Geometry check sheet. Reference: the model listing, model coordinates, mm. A direction names the side the tool comes from. Give positions to 0.01 mm unless a question says otherwise; leave off trailing zeros. Order: outer loops, then holes, each group sorted by start corner. A loop starts at its lowest first (then second) coordinate and runs counter-clockwise, first axis right, second up. Notation, with made-up numbers: M 54.25,-21 L 64.25,-21 A6 cw 64.25,-15 Z; hole C 60.25,27 d11. An arc over 180 degrees is marked long. Put each result on its own line as item: value. Start each with the question number.
Q1. Access from +Z, -Z, +X, -X, +Y, -Y to the whole of each face (thin tool, end or side, straight path). Record for faces 1 (the flat face through (-40, 0, 13)), 2 (the flat face through (-41, 25, 19.05)), 3 (the cylindrical face through (-39.92, 1.91, 23.59)), 4 (the cylindrical face through (-40.49, 48.89, -23.59)).
Q2. Go/stop test with flat-tipped pins: pin 1 (11.5 mm diameter, centred on x = -40.5, y = 18.5, fed in from -Z); pin 2 (3 mm diameter, centred on x = -23, y = 39, fed in from +Z); pin 3 (23 mm diameter, centred on x = 26.67, z = -0.23, fed in from -Y); pin 4 (6.5 mm diameter, centred on y = 27.5, z = 31.5, fed in from -X). Record where each tip stops, or that it passes through.
Q3. Material ranges on L1, parallel to Y at x = 38, z = -29; L2, parallel to Z at x = -50.5, y = 12, recorded low to high.
Q4. Section check B-B on x = 26.67. Record the cut outline in (y, z), then the cut area to 3 significant figures.
Q5. Section check D-D on x = -21.5. Record the cut outline in (y, z), then the cut area to 3 significant figures.
Q6. Mould release check, pull along Z, two halves, no side actions. Record for faces 5 (the flat face through (-40, 50.8, -13)), 6 (the flat face through (-0.4, 26.8, 38.1)), 7 (the cylindrical face through (13.982, 56.471, 0.333)): +Z half, -Z half, draft (parallel to the pull), parting line (faces both ways), or undercut.
Q7. Section check A-A on y = 14. Record the cut outline in (x, z).
Q8. Section check C-C on z = 31. Record the cut outline in (x, y), then the cut area to 3 significant figures.
```python
from build123d import *

# Parameters (mm, degrees)
F1_DEPTH      = 38.1
F2_R          = 12.7
F3_DEPTH      = 59.6909986267
F3_DEPTH_BACK = 25.4
F4_W          = 38.0999967456
F4_H          = 38.0999967456
F5_DEPTH      = 76.2
F6_R          = 12.7
F7_DEPTH      = 59.6909987267


with BuildPart() as f1:
    # F0 (on Top) → F1 (new body, symmetric)
    with BuildSketch(Plane.XY):
        with BuildLine():
            Line((46.99, 59.6899986267), (6.35, 59.6899986267))
            ThreePointArc((6.35, 59.6899986267), (-2.63025515, 55.97025515), (-6.3499986267, 46.99))
            Line((-6.3499986267, 46.99), (-6.3499986267, 6.35))
            ThreePointArc((-6.3499986267, 6.35), (-2.63025515, -2.63025515), (6.35, -6.3499986267))
            Line((6.35, -6.3499986267), (46.99, -6.3499986267))
            ThreePointArc((46.99, -6.3499986267), (55.97025515, -2.63025515), (59.6899986267, 6.35))
            Line((59.6899986267, 6.35), (59.6899986267, 46.99))
            ThreePointArc((59.6899986267, 46.99), (55.97025515, 55.97025515), (46.99, 59.6899986267))
        make_face()
        with BuildLine():
            Line((46.99, 0), (6.35, 0))
            ThreePointArc((6.35, 0), (1.8598719395, 1.8598719395), (0, 6.35))
            Line((0, 6.35), (0, 46.99))
            ThreePointArc((0, 46.99), (1.8598719395, 51.4801280605), (6.35, 53.34))
            Line((6.35, 53.34), (46.99, 53.34))
            ThreePointArc((46.99, 53.34), (51.4801280605, 51.4801280605), (53.34, 46.99))
            Line((53.34, 46.99), (53.34, 6.35))
            ThreePointArc((53.34, 6.35), (51.4801280605, 1.8598719395), (46.99, 0))
        make_face(mode=Mode.SUBTRACT)
    extrude(amount=F1_DEPTH, both=True)

    # F2 (on Front) → F3 (cut, two sides)
    with BuildSketch(Plane.XZ) as f3_sk:
        with Locations((26.67, -0.2257099867)):
            Circle(F2_R)
    extrude(amount=-F3_DEPTH, mode=Mode.SUBTRACT)
    extrude(f3_sk.sketch, amount=F3_DEPTH_BACK, mode=Mode.SUBTRACT)

    # F4 (on Right) → F5 (join)
    with BuildSketch(Plane.YZ):
        with BuildLine():
            ThreePointArc((50.8, 19.05), (48.9401280605, 23.5401280605), (44.45, 25.4))
            Line((44.45, 25.4), (6.35, 25.4))
            ThreePointArc((6.35, 25.4), (1.8598719395, 23.5401280605), (0, 19.05))
            Line((0, 19.05), (0, -19.05))
            ThreePointArc((0, -19.05), (1.8598719395, -23.5401280605), (6.35, -25.4))
            Line((6.35, -25.4), (44.45, -25.4))
            ThreePointArc((44.45, -25.4), (48.9401280605, -23.5401280605), (50.8, -19.05))
            Line((50.8, -19.05), (50.8, 19.05))
        make_face()
        with Locations((25.4, 0)):
            Rectangle(F4_W, F4_H, mode=Mode.SUBTRACT)
    extrude(amount=-F5_DEPTH)

    # F6 (on Front) → F7 (cut, through all)
    with BuildSketch(Plane.XZ):
        with Locations((-40.4242605212, 0)):
            Circle(F6_R)
    extrude(amount=-F7_DEPTH, mode=Mode.SUBTRACT)


solid = f1.part
```
Results found:
1. face 1: +Z, -Z, -X, -Y
1. face 2: -X
1. face 3: +Z, -X, -Y
1. face 4: -Z, -X, +Y
2. pin 1: stops at z = -25.4
2. pin 2: stops at z = 25.4
2. pin 3: passes through
2. pin 4: stops at x = -6.35
3. L1: y = -6.35 to 0, 53.34 to 59.69
3. L2: z = -25.4 to -19.05, 19.05 to 25.4
4. outline: M -6.35,-38.1 L 0,-38.1 L 0,-12.93 L -6.35,-12.93 Z; M -6.35,12.47 L 0,12.47 L 0,38.1 L -6.35,38.1 Z; M 53.34,-38.1 L 59.69,-38.1 L 59.69,-12.93 L 53.34,-12.93 Z; M 53.34,12.47 L 59.69,12.47 L 59.69,38.1 L 53.34,38.1 Z
4. area: 645 mm^2
5. outline: M 0,-19.05 A6.35 ccw 6.35,-25.4 L 44.45,-25.4 A6.35 ccw 50.8,-19.05 L 50.8,19.05 A6.35 ccw 44.45,25.4 L 6.35,25.4 A6.35 ccw 0,19.05 Z; hole M 6.35,-19.05 L 44.45,-19.05 L 44.45,19.05 L 6.35,19.05 Z
5. area: 1,090 mm^2
6. face 5: draft
6. face 6: +Z half
6. face 7: undercut
7. outline: M -76.2,-25.4 L -6.35,-25.4 L -6.35,-38.1 L 0,-38.1 L 0,38.1 L -6.35,38.1 L -6.35,25.4 L -76.2,25.4 L -76.2,19.05 L -6.35,19.05 L -6.35,-19.05 L -76.2,-19.05 Z; M 53.34,-38.1 L 59.69,-38.1 L 59.69,38.1 L 53.34,38.1 Z
8. outline: M -6.35,6.35 A12.7 ccw 6.35,-6.35 L 46.99,-6.35 A12.7 ccw 59.69,6.35 L 59.69,46.99 A12.7 ccw 46.99,59.69 L 6.35,59.69 A12.7 ccw -6.35,46.99 Z; hole M 0,6.35 A6.35 ccw 6.35,0 L 46.99,0 A6.35 ccw 53.34,6.35 L 53.34,46.99 A6.35 ccw 46.99,53.34 L 6.35,53.34 A6.35 ccw 0,46.99 Z
8. area: 1,410 mm^2
